```python
from build123d import *

# Parameters (mm, degrees)
F3_DEPTH = 7
F4_T     = -1.5


with BuildPart() as f3:
    # F2 (on Top) → F3 (new body)
    with BuildSketch(Plane.XY):
        with BuildLine():
            Line((25.307521998, -26.83281573), (36.2461487455, 6.83281573))
            ThreePointArc((36.2461487455, 6.83281573), (36.2461487455, 11.77708764), (33.3399786335, 15.77708764))
            Line((33.3399786335, 15.77708764), (4.7022820183, 36.583592135))
            ThreePointArc((4.7022820183, 36.583592135), (0, 38.11145618), (-4.7022820183, 36.583592135))
            Line((-4.7022820183, 36.583592135), (-33.3399786335, 15.77708764))
            ThreePointArc((-33.3399786335, 15.77708764), (-36.2461487455, 11.77708764), (-36.2461487455, 6.83281573))
            Line((-36.2461487455, 6.83281573), (-25.307521998, -26.83281573))
            ThreePointArc((-25.307521998, -26.83281573), (-22.401351886, -30.83281573), (-17.6990698677, -32.360679775))
            Line((-17.6990698677, -32.360679775), (17.6990698677, -32.360679775))
            ThreePointArc((17.6990698677, -32.360679775), (22.401351886, -30.83281573), (25.307521998, -26.83281573))
        make_face()
    extrude(amount=F3_DEPTH)

    # F4
    f4_openings = [f3.faces().sort_by_distance(p)[0] for p in [
        (0, 0, 7),
    ]]
    offset(amount=F4_T, openings=f4_openings)


solid = f3.part
```
Build history of the part. All positions in model axes, mm. A direction names the side the tool comes from. Give positions to 0.01 mm unless a question says otherwise; leave off trailing zeros. Loops run counter-clockwise (first coordinate to the right, second up) from the corner with the lowest first, then second, coordinate; pieces in that order, holes last. Notation, with made-up numbers: (3.25, -19.75) - (52.25, -19.75) arc R26 cw to (52.25, 1.25) - close; hole circle Ø3 at (45, 56). An arc over 180 degrees is marked (long way). Use a Markdown table: item, result.
(1) Pull direction Y, two halves, no side cores. Call faces 1 (the face through (-17.94, 25.11, 4.21)), 2 (the face through (36.268, 11.71, 3.451)), 3 (the face through (30.7, -10.24, 3.45)), 4 (the face through (19.222, 26.035, 3.451)): +Y half, -Y half, draft (parallel to the pull), parting line (faces both ways), or undercut.
Taken from the geometry:
| item | result |
|---|---|
| face 1 | undercut |
| face 2 | parting line |
| face 3 | -Y half |
| face 4 | +Y half |
(2) Which spindle directions (+Z, -Z, +X, -X, +Y, -Y) get a long thin tool onto all of the face, cutting with end or side? Do faces 5 (the face through (-1, 3, 0)), 6 (the face through (-29.427, -9.301, 4.212)). Say none if no direction does.
Taken from the geometry:
| item | result |
|---|---|
| face 5 | -Z, +X, -X, +Y, -Y |
| face 6 | +Z |
(3) Drop flat-ended pins along their axis: pin 1 Ø1 at (x, y) = (2.5, 13) entering from +Z; pin 2 Ø4 at (y, z) = (-7.5, 2.5) entering from -X; pin 3 Ø2 at (y, z) = (-25, 1.5) entering from -X. Give the stop position or say it passes through.
Taken from the geometry:
| item | result |
|---|---|
| pin 1 | z = 1.5 |
| pin 2 | x = -32.24 |
| pin 3 | x = -26.23 |
(4) Band-saw the part on A-A (z = 5.5). Give the cut face in (x, y).
Taken from the geometry:
| item | result |
|---|---|
| outline | (-36.25, 6.83) - (-25.31, -26.83) arc R8 ccw to (-17.7, -32.36) - (17.7, -32.36) arc R8 ccw to (25.31, -26.83) - (36.25, 6.83) arc R8 ccw to (33.34, 15.78) - (4.7, 36.58) arc R8 ccw to (-4.7, 36.58) - (-33.34, 15.78) arc R8 ccw to start; hole (-34.82, 7.3) - (-23.88, -26.37) arc R6.5 ccw to (-17.7, -30.86) - (17.7, -30.86) arc R6.5 ccw to (23.88, -26.37) - (34.82, 7.3) arc R6.5 ccw to (32.46, 14.56) - (3.82, 35.37) arc R6.5 ccw to (-3.82, 35.37) - (-32.46, 14.56) arc R6.5 ccw to start |
(5) Band-saw the part on B-B (y = 9). Give the cut face in (x, z), and give its area (3 significant figures).
Taken from the geometry:
| item | result |
|---|---|
| outline | (-36.63, 0) - (36.63, 0) - (36.63, 7) - (35.13, 7) - (35.13, 1.5) - (-35.13, 1.5) - (-35.13, 7) - (-36.63, 7) - close |
| area | 126 mm2 |
(6) Wall check: line 1 along Z through (x, y) = (-1, 8.5); line 2 along Y through (x, z) = (17, 6.75); line 3 along X through (y, z) = (0.5, 3.75). Give the ranges that are in metal, low to high.
Taken from the geometry:
| item | result |
|---|---|
| line 1 | 0 to 1.5 |
| line 2 | -32.36 to -30.86, 25.79 to 27.65 |
| line 3 | -34.19 to -32.61, 32.61 to 34.19 |
(7) Band-saw the part on C-C (x = 21). Give the cut face in (y, z).
Taken from the geometry:
| item | result |
|---|---|
| outline | (-31.65, 0) - (24.74, 0) - (24.74, 7) - (22.89, 7) - (22.89, 1.5) - (-29.96, 1.5) - (-29.96, 7) - (-31.65, 7) - close |
